Geometry check sheet. Reference: the model listing, model coordinates, mm. Face numbers are marked on the shaded views. A direction names the side the tool comes from. Coordinates: 2 decimals unless noted, no trailing zeros.
from build123d import *

# Parameters (mm, degrees)
F0_R     = 30
F0_R_2   = 2
F0_R_3   = 19.5
F1_DEPTH = 3
F0_R_4   = 12.5
F2_DEPTH = 3.5
F3_SIZE  = 0.5
F4_SIZE  = 0.25


with BuildPart() as f1:
    # F0 (on Right) → F1 (new body, symmetric)
    with BuildSketch(Plane.YZ):
        Circle(F0_R)
        with Locations((-17.67767, -17.67767)):
            Circle(F0_R_2, mode=Mode.SUBTRACT)
        with Locations((0, -25)):
            Circle(F0_R_2, mode=Mode.SUBTRACT)
        with Locations((17.67767, -17.67767)):
            Circle(F0_R_2, mode=Mode.SUBTRACT)
        with Locations((-25, 0)):
            Circle(F0_R_2, mode=Mode.SUBTRACT)
        with Locations((-17.67767, 17.67767)):
            Circle(F0_R_2, mode=Mode.SUBTRACT)
        Circle(F0_R_3, mode=Mode.SUBTRACT)
        with Locations((25, 0)):
            Circle(F0_R_2, mode=Mode.SUBTRACT)
        with Locations((0, 25)):
            Circle(F0_R_2, mode=Mode.SUBTRACT)
        with Locations((17.67767, 17.67767)):
            Circle(F0_R_2, mode=Mode.SUBTRACT)
    extrude(amount=F1_DEPTH, both=True)

    # F0 (on Right) → F2 (join, symmetric)
    with BuildSketch(Plane.YZ):
        Circle(F0_R_3)
        Circle(F0_R_4, mode=Mode.SUBTRACT)
    extrude(amount=F2_DEPTH, both=True)

    # F3
    f3_edges = [f1.edges().sort_by_distance(p)[0] for p in [
        (3.5, -12.5, 0),
        (0, 12.5, 0),
        (-3.5, -12.5, 0),
    ]]
    chamfer(f3_edges, length=F3_SIZE)

    # F4
    f4_edges = [f1.edges().sort_by_distance(p)[0] for p in [
        (-3, -30, 0),
        (0, 30, 0),
        (3, -30, 0),
    ]]
    chamfer(f4_edges, length=F4_SIZE)


solid = f1.part
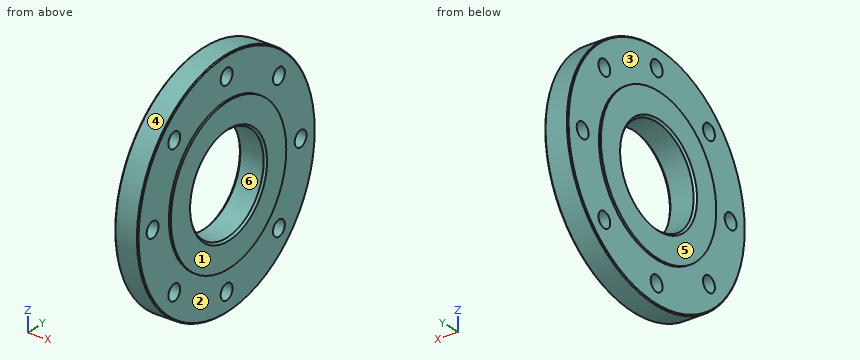
(1) Sectioned sample at A-A on y = 0. State how many separate pieces and enclosed holes the cut face has, and give its area (3 significant figures).
Findings:
separate pieces: 4
enclosed holes: 0
area: 175 mm2
(2) Draft check along Z on the marked faces 4, 5 and 6. Enter one of: +Z half, -Z half, draft (parallel to the pull), parting line (faces both ways), or undercut.
Findings:
face 4: parting line
face 5: draft
face 6: undercut
(3) Access from +Z, -Z, +X, -X, +Y, -Y to the whole of each face (thin tool, end or side, straight path). Record for the marked faces 1, 2 and 3.
Findings:
face 1: +Z, -Z, +X, +Y, -Y
face 2: +X
face 3: -X
(4) Scan lines: L1, parallel to Z at x = 2, y = 19.5; L2, parallel to Z at x = 3.25, y = -0.5; L3, parallel to Z at x = -0.5, y = 10.5. Record each from-to range of solid material in increasing order.
Findings:
L1: z = -22.8 to -18.5, -16.85 to 16.85, 18.5 to 22.8
L2: z = -19.49 to -12.74, 12.74 to 19.49
L3: z = -28.1 to -6.78, 6.78 to 28.1
(5) Gauge pin test, flat ends, axial feed: pin 1 Ø2.5 at (y, z) = (17.68, 17.68) entering from -X; pin 2 Ø1 at (x, z) = (-2.5, 17.5) entering from +Y; pin 3 Ø5 at (y, z) = (17.68, -17.68) entering from -X; pin 4 Ø1.5 at (x, y) = (2.5, 10) entering from +Z. Record the tip position at first contact, or that the pin passes through.
Findings:
pin 1: passes through
pin 2: stops at y = 24.72
pin 3: stops at x = -3
pin 4: stops at z = 28.54
